Source: CAD feature listing. Evaluate the final solid. Frame: model axes, mm. Face numbers are marked on the shaded views. A direction names the side the tool comes from. Give positions to 0.01 mm unless a question says otherwise; leave off trailing zeros. Loops run counter-clockwise (first coordinate to the right, second up) from the corner with the lowest first, then second, coordinate; pieces in that order, holes last. Notation, with made-up numbers: (68.5, -16) -> (87.5, -16) arc R31 cw to (87.5, 12) -> close; hole circle Ø2 at (50.25, 16.5). An arc over 180 degrees is marked (long way). Answer as a JSON object with one key per item and string values. Group by question number.
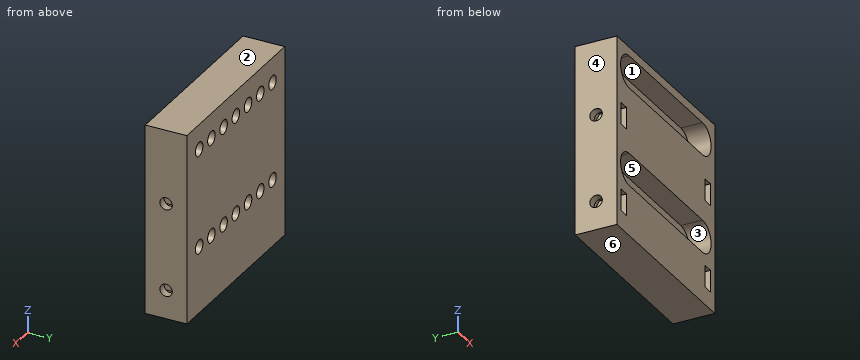
Autodesk Inventor part; units mm, degrees
ref_plane "YZ Plane" through (0, 0, 0) normal (1, 0, 0) x (0, 1, 0)
ref_plane "XZ Plane" through (0, 0, 0) normal (0, 1, 0) x (-1, 0, 0)
ref_plane "XY Plane" through (0, 0, 0) normal (0, 0, 1) x (1, 0, 0)
sketch "Sketch1" plane through (0, 0, 0) normal (0, 1, 0) x (-1, 0, 0)
  line L0 (-25.4, 20.32) -> (-25.4, -31.75)
  line L1 (-25.4, -31.75) -> (25.4, -31.75)
  line L2 (25.4, -31.75) -> (25.4, 20.32)
  line L3 (25.4, 31.75) -> (-25.4, -31.75) construction
  line L4 (-25.4, 31.75) -> (25.4, -31.75) construction
  line L5 (15.875, 13.4747) -> (-15.875, 13.4747) construction
  line L6 (-15.875, -13.4747) -> (15.875, -13.4747) construction
  line L7 (25.4, 20.32) -> (-25.4, 20.32)
  circle A0 centre (0, 13.4747) radius 1.9304
  circle A1 centre (0, -13.4747) radius 1.9304
  circle A2 centre (6.35, 13.4747) radius 1.9304
  circle A3 centre (6.35, -13.4747) radius 1.9304
  circle A4 centre (12.7, 13.4747) radius 1.9304
  circle A5 centre (12.7, -13.4747) radius 1.9304
  circle A6 centre (19.05, 13.4747) radius 1.9304
  circle A7 centre (19.05, -13.4747) radius 1.9304
  circle A8 centre (-6.35, -13.4747) radius 1.9304
  circle A9 centre (-6.35, 13.4747) radius 1.9304
  circle A10 centre (-12.7, -13.4747) radius 1.9304
  circle A11 centre (-12.7, 13.4747) radius 1.9304
  circle A12 centre (-19.05, -13.4747) radius 1.9304
  circle A13 centre (-19.05, 13.4747) radius 1.9304
  point P0 (0, 0)
  dimension "d0" = 50.8
  dimension "d2" = 26.9494
  dimension "d3" = 13.4747
  dimension "d4" = 26.9494
  dimension "d7" = 9.525
  dimension "d49" = 6.8453
  dimension "d50" = 3.8608
  dimension "d51" = 3.8608
  dimension "d54" = 6.35
  dimension "d64" = 6.35
extrude "Extrusion1" add sketch "Sketch1" along normal blind 11.43
sketch "Sketch3" plane through (0, 0, 0) normal (0, -1, 0) x (1, 0, 0)
  line L0 (-15.875, -13.4747) -> (15.875, -13.4747) construction
  line L1 (-15.875, 13.4747) -> (15.875, 13.4747) construction
  circle A0 centre (19.05, 13.4747) radius 1.9304
  arc A1 (19.05, 9.0297) -> (19.05, 17.9197) centre (19.05, 13.4747) ccw
  circle A2 centre (-19.05, 13.4747) radius 1.9304
  arc A3 (-19.05, 17.9197) -> (-19.05, 9.0297) centre (-19.05, 13.4747) ccw
  line L2 (-19.05, 17.9197) -> (19.05, 17.9197)
  line L3 (-19.05, 9.0297) -> (19.05, 9.0297)
  circle A4 centre (19.05, -13.4747) radius 1.9304
  arc A5 (19.05, -17.9197) -> (19.05, -9.0297) centre (19.05, -13.4747) ccw
  circle A6 centre (-19.05, -13.4747) radius 1.9304
  arc A7 (-19.05, -9.0297) -> (-19.05, -17.9197) centre (-19.05, -13.4747) ccw
  line L4 (-19.05, -9.0297) -> (19.05, -9.0297)
  line L5 (-19.05, -17.9197) -> (19.05, -17.9197)
  point P0 (0, 0)
  point P1 (0, -13.4747)
  point P2 (0, 13.4747)
  dimension "d66" = 8.89
  dimension "d67" = 8.89
  dimension "d68" = 8.89
  dimension "d69" = 8.89
extrude "Extrusion3" cut sketch "Sketch3" against normal blind 5.9436
ref_plane "Work Plane2" through (-20.4, 0, -31.75) normal (-1, 0, 0) x (0, 0, 1)
sketch "Sketch5" plane through (-20.4, 0, -31.75) normal (-1, 0, 0) x (0, 0, 1)
  circle A0 centre (31.75, 5.715) radius 3.45 construction
  line L0 (52.07, 0) -> (0, 0)
  line L1 (52.07, 11.43) -> (0, 11.43)
  line L2 (0, 0) -> (0, 11.43)
  line L3 (28.7622, 0) -> (28.7622, 7.44)
  line L4 (28.7622, 7.44) -> (31.75, 9.165)
  line L5 (31.75, 9.165) -> (34.7378, 7.44)
  line L6 (34.7378, 7.44) -> (34.7378, 0)
  line L7 (28.7622, 0) -> (34.7378, 0)
  line L8 (13.8303, 0) -> (13.8303, 5.9436) construction
  line L9 (49.6697, 0) -> (49.6697, 5.9436) construction
  circle A1 centre (7.8403, 5.715) radius 3.45 construction
  line L10 (4.8525, 0) -> (4.8525, 7.44)
  line L11 (4.8525, 7.44) -> (7.8403, 9.165)
  line L12 (7.8403, 9.165) -> (10.8281, 7.44)
  line L13 (10.8281, 7.44) -> (10.8281, 0)
  line L14 (4.8525, 0) -> (10.8281, 0)
  circle A2 centre (7.8403, 5.715) radius 1.7
  circle A3 centre (31.75, 5.715) radius 1.7
  point P0 (31.75, 0)
  dimension "d24" = 6.9
  dimension "d26" = 5.715
  dimension "d29" = 6.9
  dimension "d31" = 5.99
  dimension "d33" = 5.715
  dimension "d37" = 3.4
  dimension "d38" = 3.4
  dimension "d48" = 31.75
extrude "Extrusion4" cut sketch "Sketch5" along normal blind 2.8 contours L0 L10 L11 L12 L13 | L0 L3 L4 L5 L6 | A2 | A3
sketch "Sketch6" plane through (-25.4, 0, -31.75) normal (-1, 0, 0) x (0, 0, 1)
  circle A0 centre (7.8403, 5.715) radius 1.7
  circle A1 centre (31.75, 5.715) radius 1.7
  line L0 (13.8303, 0) -> (13.8303, 5.9436)
  line L1 (63.5, 0) -> (63.5, 11.43)
  line L2 (49.6697, 0) -> (49.6697, 5.9436)
  point P0 (31.75, 0)
  dimension "d40" = 3.4
  dimension "d41" = 3.4
  dimension "d43" = 5.99
extrude "Extrusion5" cut sketch "Sketch6" against normal blind 6
ref_plane "Work Plane3" through (0, 0, -31.75) normal (-1, 0, 0) x (0, 0, 1)
mirror "Mirror1" about plane through (0, 0, -31.75) normal (-1, 0, 0) of "Extrusion4"
mirror "Mirror2" about plane through (0, 0, -31.75) normal (-1, 0, 0) of "Extrusion5"
sketch "Sketch7" plane through (0, 0, 0) normal (0, -1, 0) x (1, 0, 0)
  point P0 (0, 0)
equation "\"d4\" = d2"
equation "\"d26\" = 0.5 * d25"
equation "\"d33\" = d26"
equation "\"d43\" = d31"
properties part number "driven wheel mount to xrail adjustable holes"
(1) Mould query, pull axis X, two halves, no side actions, for the marked faces 3, 4, 5 and 6. Classes: pulls with the +X half, pulls with the -X half, needs draft (parallel to the pull), parting line crosses it, or undercut.
(2) Access query for the marked faces 1 and 2. Directions: +Z, -Z, +X, -X, +Y, -Y. A direction counts if a zero-diameter tool reaches every point of the face in a straight line with its end or side. Return the directions, or none.
(3) Material intervals for line 1 (Z direction, x = 6.35, y = 9.75); line 2 (Z direction, x = 5, y = 2.25); line 3 (X direction, y = 3, z = -22), sorted ascending. Write a range as from..to.
(4) First-contact query: pin 1 (2 mm diameter, centred on y = 5.72, z = -23.91, fed in from +X); pin 2 (2.5 mm diameter, centred on x = -19.05, z = 13.47, fed in from -Y); pin 3 (3 mm diameter, centred on y = 5.72, z = -23.91, fed in from -X); pin 4 (6 mm diameter, centred on x = 19.05, z = 13.47, fed in from -Y). Flat tips, straight axial feed; report the tip coordinate or a pass-through.
(5) Section query A-A on y = 1.75. State how many separate pieces and enclosed holes the cut face has, plus the area to 3 significant figures.
(6) Section query B-B on x = -1. Return the cut outline in (y, z), plus the area to 3 significant figures.
(7) Section query C-C on x = -16.5. Return the cut outline in (y, z).
Result:
{
 "1": {"face 3": "undercut", "face 4": "pulls with the -X half", "face 5": "undercut", "face 6": "needs draft"},
 "2": {"face 1": "-Y", "face 2": "+Z, +X, -X, +Y, -Y"},
 "3": {"line 1": "-31.75..-15.41, -11.54..11.54, 15.41..20.32", "line 2": "-31.75..-17.92, -9.03..9.03, 17.92..20.32", "line 3": "-25.4..-23.2, -20.4..20.4, 23.2..25.4"},
 "4": {"pin 1": "x = 19.4", "pin 2": "through", "pin 3": "x = -19.4", "pin 4": "y = 5.94"},
 "5": {"separate pieces": "1", "enclosed holes": "6", "area": "1,780 mm²"},
 "6": {"outline": "(0, -31.75) -> (11.43, -31.75) -> (11.43, -15.13) -> (5.94, -15.13) -> (5.94, -17.92) -> (0, -17.92) -> close; (0, -9.03) -> (5.94, -9.03) -> (5.94, -11.82) -> (11.43, -11.82) -> (11.43, 11.82) -> (5.94, 11.82) -> (5.94, 9.03) -> (0, 9.03) -> close; (0, 17.92) -> (5.94, 17.92) -> (5.94, 15.13) -> (11.43, 15.13) -> (11.43, 20.32) -> (0, 20.32) -> close", "area": "453 mm²"},
 "7": {"outline": "(0, -31.75) -> (11.43, -31.75) -> (11.43, 20.32) -> (0, 20.32) -> (0, 17.92) -> (5.94, 17.92) -> (5.94, 9.03) -> (0, 9.03) -> (0, -9.03) -> (5.94, -9.03) -> (5.94, -17.92) -> (0, -17.92) -> close"}
}
